Can you work these out from the drawing? Everything is in mm from the part's minimum corner. A direction names the side the tool comes from. Round coordinates to 2 decimals unless told otherwise and drop trailing zeros. Loops run counter-clockwise (first coordinate to the right, second up) from the corner with the lowest first, then second, coordinate; pieces in that order, holes last. Notation, with made-up numbers: (23, 0) -> (46, 0) arc R21 cw to (46, 25) -> close; hole circle Ø7 at (66, 22.5). An arc over 180 degrees is marked (long way). One line per item, written item: value.
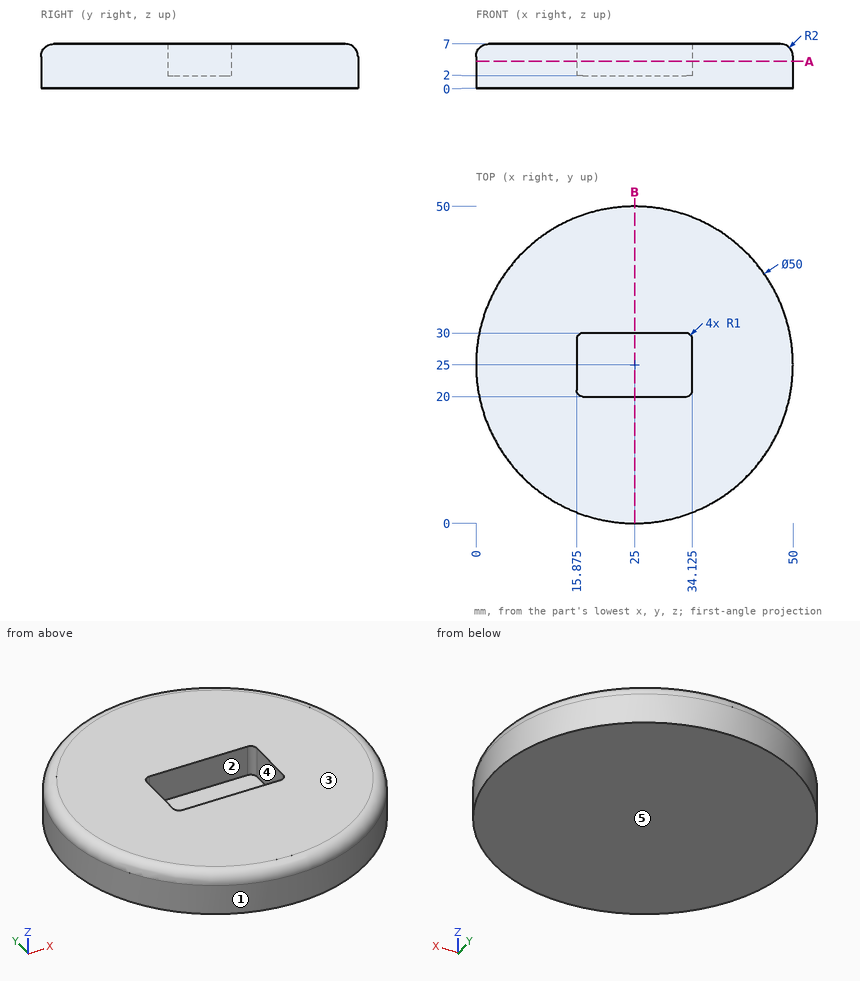
(1) Please list where these lines run through material, in increasing order: L1, parallel to X at y = 25.5, z = 3.5 (3 decimals); L2, parallel to X at y = 24.5, z = 0.5 (3 decimals); L3, parallel to Y at x = 26.5, z = 2.5.
Results below:
L1: x = 0.005 to 15.875, 34.125 to 49.995
L2: x = 0.005 to 49.995
L3: y = 0.05 to 20, 30 to 49.95
(2) On a 3-axis mill with a long thin cutter (end or side, diameter ignored), from which of +Z, -Z, +X, -X, +Y, -Y can I reach the whole of each face in a straight line? I mean the marked faces 4 and 5. Say none if no direction works.
Results below:
face 4: +Z
face 5: -Z, +X, -X, +Y, -Y
(3) Imagine slicing it at A-A on z = 4.25. Write out the boundary of the cut face in (x, y) (3 decimals).
Results below:
outline: circle Ø50 at (25, 25); hole (15.875, 21) arc R1 ccw to (16.875, 20) -> (33.125, 20) arc R1 ccw to (34.125, 21) -> (34.125, 29) arc R1 ccw to (33.125, 30) -> (16.875, 30) arc R1 ccw to (15.875, 29) -> close
(4) We'd pull the mould along Y, two halves only. Please class the marked faces 1, 2 and 3: +Y half, -Y half, draft (parallel to the pull), parting line (faces both ways), or undercut.
Results below:
face 1: parting line
face 2: undercut
face 3: draft
(5) For pin 1 Ø3 at (y, z) = (22, 2.5) entering from +X; pin 2 Ø8 at (x, y) = (27, 25.5) entering from +Z; pin 3 Ø1.5 at (y, z) = (11.5, 1) entering from -X, each with a flat end and sliding along its axis, tell me the tip position at first contact or that it passes through.
Results below:
pin 1: stops at x = 49.95
pin 2: stops at z = 2
pin 3: stops at x = 3.5
(6) Imagine slicing it at B-B on x = 25. Write out the boundary of the cut face in (y, z).
Results below:
outline: (0, 0) -> (50, 0) -> (50, 5) arc R2 ccw to (48, 7) -> (30, 7) -> (30, 2) -> (20, 2) -> (20, 7) -> (2, 7) arc R2 ccw to (0, 5) -> close
